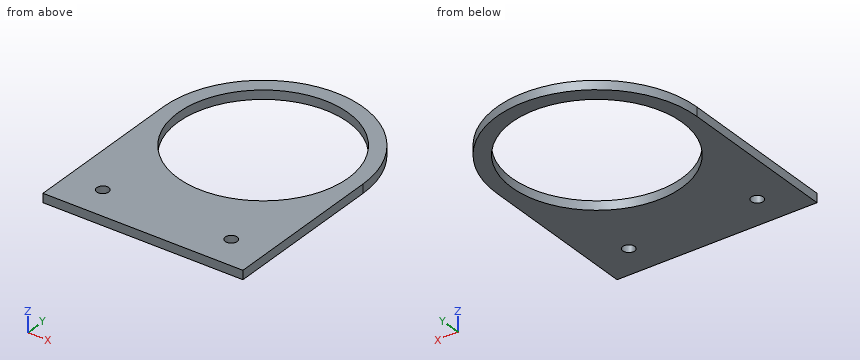
```python
from build123d import *

# Parameters (mm, degrees)
SKETCH1_R           = 28.5
SKETCH1_R_2         = 2
BOSS_EXTRUDE1_DEPTH = 3


with BuildPart() as part:
    # Sketch1 → Boss-Extrude1 (new body)
    with BuildSketch(Plane.XY):
        with BuildLine():
            Line((-33.5, 0), (33.5, 0))
            Line((33.5, 0), (33.5, 55))
            ThreePointArc((33.5, 55), (0, 88.5), (-33.5, 55))
            Line((-33.5, 55), (-33.5, 0))
        make_face()
        with Locations((0, 55)):
            Circle(SKETCH1_R, mode=Mode.SUBTRACT)
        with Locations((-21.5, 11)):
            Circle(SKETCH1_R_2, mode=Mode.SUBTRACT)
        with Locations(Location((21.5, 11, 0), (0, 0, 180))):
            Circle(SKETCH1_R_2, mode=Mode.SUBTRACT)
    extrude(amount=BOSS_EXTRUDE1_DEPTH)


solid = part.part
```
Design review of the part built by this model. Coordinates are the model's own, in mm. Give positions to 0.01 mm unless a question says otherwise; leave off trailing zeros. Order: outer loops, then holes, each group sorted by start corner. A loop starts at its lowest first (then second) coordinate and runs counter-clockwise, first axis right, second up. Notation, with made-up numbers: (30.5, 75.5) - (63.5, 75.5) arc R20 cw to (63.5, 96.5) - close; hole circle Ø8 at (-5, 43). An arc over 180 degrees is marked (long way). Use a Markdown table: item, result. Add a question column.
(1) Add section C-C on z = 1.05. Give the boundary of the cut face in (x, y).
(2) Add section A-A on y = 11. Give the boundary of the cut face in (x, z), then the cut area to 3 significant figures.
(3) Wall thickness on probe 1 along Y at (x, z) = (21.5, 1.65); probe 2 along Y at (x, z) = (21, 1.55); probe 3 along Y at (x, z) = (0, 0.9): over which ranges is each line inside the solid? List them lowest first. Write a range as [from, to].
(4) Add section D-D on x = -21.5. Give the boundary of the cut face in (y, z).
(5) Add section B-B on x = 27. Give the boundary of the cut face in (y, z).
Report:
| question | item | result |
|---|---|---|
| 1 | outline | (-33.5, 0) - (33.5, 0) - (33.5, 55) arc R33.5 ccw to (-33.5, 55) - close; hole circle Ø57 at (0, 55); hole circle Ø4 at (-21.5, 11); hole circle Ø4 at (21.5, 11) |
| 2 | outline | (-33.5, 0) - (-23.5, 0) - (-23.5, 3) - (-33.5, 3) - close; (-19.5, 0) - (19.5, 0) - (19.5, 3) - (-19.5, 3) - close; (23.5, 0) - (33.5, 0) - (33.5, 3) - (23.5, 3) - close |
| 2 | area | 177 mm² |
| 3 | probe 1 | y = [0, 9], [13, 36.29], [73.71, 80.69] |
| 3 | probe 2 | y = [0, 9.06], [12.94, 35.73], [74.27, 81.1] |
| 3 | probe 3 | y = [0, 26.5], [83.5, 88.5] |
| 4 | outline | (0, 0) - (9, 0) - (9, 3) - (0, 3) - close; (13, 0) - (36.29, 0) - (36.29, 3) - (13, 3) - close; (73.71, 0) - (80.69, 0) - (80.69, 3) - (73.71, 3) - close |
| 5 | outline | (0, 0) - (45.88, 0) - (45.88, 3) - (0, 3) - close; (64.12, 0) - (74.83, 0) - (74.83, 3) - (64.12, 3) - close |
